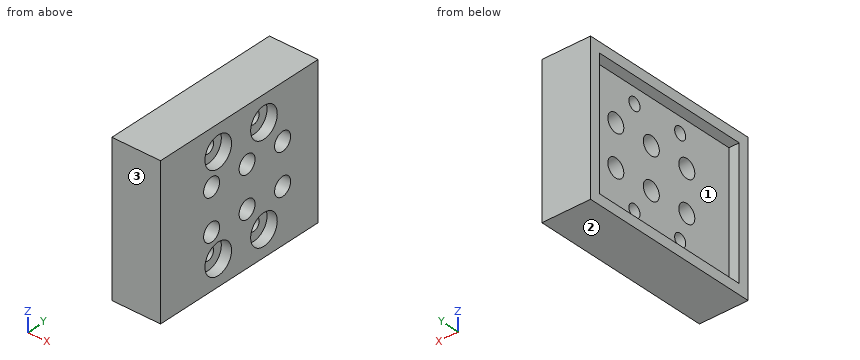
```python
from build123d import *

# Parameters (mm, degrees)
SKETCH_1_W          = 25
SKETCH_1_H          = 31.5
EXTRUDE_1_DEPTH     = 2
SKETCH_2_R          = 1.25
CUT_EXTRUDE_1_DEPTH = 5
SKETCH_3_W          = 2
SKETCH_3_H          = 31.5
EXTRUDE_2_DEPTH     = 2
SKETCH_4_W          = 2
SKETCH_4_H          = 31.5
EXTRUDE_3_DEPTH     = 2
SKETCH_5_W          = 2
SKETCH_5_H          = 31.5
EXTRUDE_4_DEPTH     = 2
SKETCH_6_W          = 2
SKETCH_6_H          = 31.5
EXTRUDE_5_DEPTH     = 2
SKETCH_7_W          = 4
SKETCH_7_H          = 29
EXTRUDE_6_DEPTH     = 2
SKETCH_8_W          = 4
SKETCH_8_H          = 29
EXTRUDE_7_DEPTH     = 2
EXTRUDE_START       = 3
SKETCH_9_W          = 29
SKETCH_9_H          = 35.5
SKETCH_9_R          = 1.25
EXTRUDE_8_DEPTH     = 3
EXTRUDE_START_2     = 2.5
SKETCH_11_W         = 29
SKETCH_11_H         = 35.5
SKETCH_11_R         = 1.25
EXTRUDE_9_DEPTH     = 2.5
SKETCH_12_R         = 1.8
CUT_EXTRUDE_2_DEPTH = 13.5
SKETCH_13_R         = 3
CUT_EXTRUDE_3_DEPTH = 2


with BuildPart() as part:
    # 草圖1 → 填料-伸長1 (new body)
    with BuildSketch(Plane(origin=(0, 0, 0), x_dir=(0, 0, -1), z_dir=(1, 0, 0))):
        with Locations((12.5, 15.75)):
            Rectangle(SKETCH_1_W, SKETCH_1_H)
    extrude(amount=EXTRUDE_1_DEPTH)

    # 草圖2 → 除料-伸長1 (cut)
    with BuildSketch(Plane(origin=(2, 0, 0), x_dir=(0, 0, -1), z_dir=(1, 0, 0))):
        with Locations((22, 21.3)):
            Circle(SKETCH_2_R)
        with Locations((22, 11)):
            Circle(SKETCH_2_R)
        with Locations((3, 21.3)):
            Circle(SKETCH_2_R)
        with Locations((3, 11)):
            Circle(SKETCH_2_R)
    extrude(amount=-CUT_EXTRUDE_1_DEPTH, mode=Mode.SUBTRACT)

    # 草圖3 → 填料-伸長2 (add)
    with BuildSketch(Plane.XY):
        with Locations((1, 15.75)):
            Rectangle(SKETCH_3_W, SKETCH_3_H)
    extrude(amount=EXTRUDE_2_DEPTH)

    # 草圖4 → 填料-伸長3 (add)
    with BuildSketch(Plane(origin=(0, 0, -25), x_dir=(-1, 0, 0), z_dir=(0, 0, -1))):
        with Locations((-1, 15.75)):
            Rectangle(SKETCH_4_W, SKETCH_4_H)
    extrude(amount=EXTRUDE_3_DEPTH)

    # 草圖5 → 填料-伸長4 (add)
    with BuildSketch(Plane.ZY):
        with Locations((-26, 15.75)):
            Rectangle(SKETCH_5_W, SKETCH_5_H)
    extrude(amount=EXTRUDE_4_DEPTH)

    # 草圖6 → 填料-伸長5 (add)
    with BuildSketch(Plane.ZY):
        with Locations((1, 15.75)):
            Rectangle(SKETCH_6_W, SKETCH_6_H)
    extrude(amount=EXTRUDE_5_DEPTH)

    # 草圖7 → 填料-伸長6 (add)
    with BuildSketch(Plane(origin=(0, 31.5, 0), x_dir=(1, 0, 0), z_dir=(0, 1, 0))):
        with Locations((0, 12.5)):
            Rectangle(SKETCH_7_W, SKETCH_7_H)
    extrude(amount=EXTRUDE_6_DEPTH)

    # 草圖8 → 填料-伸長7 (add)
    with BuildSketch(Plane(origin=(0, 0, 0), x_dir=(-1, 0, 0), z_dir=(0, -1, 0))):
        with Locations((0, 12.5)):
            Rectangle(SKETCH_8_W, SKETCH_8_H)
    extrude(amount=EXTRUDE_7_DEPTH)

    # 草圖9 → 填料-伸長8 (add)
    with BuildSketch(Plane(origin=(2, 0, 0), x_dir=(0, 0, -1), z_dir=(1, 0, 0)).offset(EXTRUDE_START)):
        with Locations((12.5, 15.75)):
            Rectangle(SKETCH_9_W, SKETCH_9_H)
        with Locations((3, 21.3)):
            Circle(SKETCH_9_R, mode=Mode.SUBTRACT)
        with Locations((22, 21.3)):
            Circle(SKETCH_9_R, mode=Mode.SUBTRACT)
        with Locations((22, 11)):
            Circle(SKETCH_9_R, mode=Mode.SUBTRACT)
        with Locations((3, 11)):
            Circle(SKETCH_9_R, mode=Mode.SUBTRACT)
    extrude(amount=-EXTRUDE_8_DEPTH)

    # 草圖11 → 填料-伸長9 (add)
    with BuildSketch(Plane(origin=(5, 0, 0), x_dir=(0, 0, -1), z_dir=(1, 0, 0)).offset(EXTRUDE_START_2)):
        with Locations((12.5, 15.75)):
            Rectangle(SKETCH_11_W, SKETCH_11_H)
        with Locations((3, 21.3)):
            Circle(SKETCH_11_R, mode=Mode.SUBTRACT)
        with Locations((22, 21.3)):
            Circle(SKETCH_11_R, mode=Mode.SUBTRACT)
        with Locations((22, 11)):
            Circle(SKETCH_11_R, mode=Mode.SUBTRACT)
        with Locations((3, 11)):
            Circle(SKETCH_11_R, mode=Mode.SUBTRACT)
    extrude(amount=-EXTRUDE_9_DEPTH)

    # 草圖12 → 除料-伸長2 (cut)
    with BuildSketch(Plane(origin=(7.5, 0, 0), x_dir=(0, 0, -1), z_dir=(1, 0, 0))):
        with Locations((8.5, 25.5)):
            Circle(SKETCH_12_R)
        with Locations((16.5, 25.5)):
            Circle(SKETCH_12_R)
        with Locations((16.5, 17.5)):
            Circle(SKETCH_12_R)
        with Locations((16.5, 9.5)):
            Circle(SKETCH_12_R)
        with Locations((8.5, 9.5)):
            Circle(SKETCH_12_R)
        with Locations((8.5, 17.5)):
            Circle(SKETCH_12_R)
    extrude(amount=-CUT_EXTRUDE_2_DEPTH, mode=Mode.SUBTRACT)

    # 草圖13 → 除料-伸長3 (cut)
    with BuildSketch(Plane(origin=(7.5, 0, 0), x_dir=(0, 0, -1), z_dir=(1, 0, 0))):
        with Locations((3, 21.3)):
            Circle(SKETCH_13_R)
        with Locations((3, 11)):
            Circle(SKETCH_13_R)
        with Locations((22, 11)):
            Circle(SKETCH_13_R)
        with Locations((22, 21.3)):
            Circle(SKETCH_13_R)
    extrude(amount=-CUT_EXTRUDE_3_DEPTH, mode=Mode.SUBTRACT)


solid = part.part
```
The listing builds one solid part. Answer for the finished solid, in the listing's coordinates (mm). Face numbers are marked on the shaded views. Coordinates: 2 decimals unless noted, no trailing zeros. Loops run counter-clockwise (first coordinate to the right, second up) from the corner with the lowest first, then second, coordinate; pieces in that order, holes last. Notation, with made-up numbers: M 50.25,-19.75 L 83.25,-19.75 A13 cw 83.25,2.25 Z; hole C -14,20 d8. An arc over 180 degrees is marked long. Answer as CSV lines item,"result". Start each with the question number.
(1) The part is cut by section B-B (x = 1.75). State how many separate pieces and enclosed holes the cut face has, and give its area (3 significant figures).
(2) The mould has two halves that part along Y. Classify the marked faces 1, 2 and 3: pulls with the +Y half, pulls with the -Y half, needs draft (parallel to the pull), parting line crosses it, or undercut.
(3) The part is cut by section D-D (z = -15.75). Give the vertices of the cut face in (x, y).
(4) Given pin 1 (9.5 mm diameter, centred on y = 11, z = -22, fed in from +X); pin 2 (6 mm diameter, centred on y = 17.5, z = -16.5, fed in from -X); pin 3 (1.8 mm diameter, centred on y = 11.5, z = -3.5, fed in from +X), each flat-ended and moving along its own axis, determine where each tip first touches the part or whether it passes through.
(5) The part is cut by section A-A (y = 21.3). Give the vertices of the cut face in (x, z).
(6) Find the intervals of material crossed by L1, parallel to Y at x = 6.2, z = -3; L2, parallel to Y at x = 6, z = -16.5; L3, parallel to Z at x = 6, y = 26.5, in increasing order. Write a range as [from, to].
(7) The part is cut by section C-C (z = -22). Give the vertices of the cut face in (x, y).
Determined:
1,separate pieces,"1"
1,enclosed holes,"10"
1,area,"949 mm2"
2,face 1,"undercut"
2,face 2,"needs draft"
2,face 3,"pulls with the -Y half"
3,outline,"M -2,-2 L 7.5,-2 L 7.5,7.86 L 0,7.86 L 0,0 L -2,0 Z; M -2,31.5 L 0,31.5 L 0,27.14 L 7.5,27.14 L 7.5,33.5 L -2,33.5 Z; M 0,11.14 L 7.5,11.14 L 7.5,15.86 L 0,15.86 Z; M 0,19.14 L 7.5,19.14 L 7.5,23.86 L 0,23.86 Z"
4,pin 1,"x = 7.5"
4,pin 2,"x = 0"
4,pin 3,"x = 5.5"
5,outline,"M -2,-27 L 7.5,-27 L 7.5,-25 L 5.5,-25 L 5.5,-23.25 L 0,-23.25 L 0,-25 L -2,-25 Z; M -2,0 L 0,0 L 0,-1.75 L 5.5,-1.75 L 5.5,0 L 7.5,0 L 7.5,2 L -2,2 Z; M 0,-20.75 L 5.5,-20.75 L 5.5,-19 L 7.5,-19 L 7.5,-6 L 5.5,-6 L 5.5,-4.25 L 0,-4.25 Z"
6,L1,"[-2, 8], [14, 18.3], [24.3, 33.5]"
6,L2,"[-2, 7.7], [11.3, 15.7], [19.3, 23.7], [27.3, 33.5]"
6,L3,"[-27, -18], [-15, -10], [-7, 2]"
7,outline,"M -2,-2 L 7.5,-2 L 7.5,8 L 5.5,8 L 5.5,9.75 L 0,9.75 L 0,0 L -2,0 Z; M -2,31.5 L 0,31.5 L 0,22.55 L 5.5,22.55 L 5.5,24.3 L 7.5,24.3 L 7.5,33.5 L -2,33.5 Z; M 0,12.25 L 5.5,12.25 L 5.5,14 L 7.5,14 L 7.5,18.3 L 5.5,18.3 L 5.5,20.05 L 0,20.05 Z"
